Answer from the drawing. Dimensions are ordinates in mm from the lowest x, y and z of the part. A direction names the side the tool comes from. Coordinates: 2 decimals unless noted, no trailing zeros. Write each loop counter-clockwise with the first axis right and the second up, starting at its lowest first coordinate (ties: lowest second). Pieces come first, ordered by that corner, then holes. Notation, with made-up numbers: (17, 16) - (56, 16) arc R16 cw to (56, 31) - close; hole circle Ø1 at (86, 8.5). An arc over 180 degrees is marked (long way). Use one line per item in the form item = value. Start each with the question number.
Item 1: A cutting plane is placed at C-C (y = 24). Write down the section's boundary in (x, z).
Item 2: A cutting plane is placed at D-D (y = 9). Write down the section's boundary in (x, z) (1 decimal).
Item 3: Consider probe 1 along Y at (x, z) = (12.7, 7.5) (1 decimal); probe 2 along Y at (x, z) = (10.25, 24.25); probe 3 along X at (y, z) = (25.4, 6) (1 decimal). Determine where each line is inside the solid, lowest interval first.
Item 4: A cutting plane is placed at A-A (x = 12.7). Write down the section's boundary in (y, z) (1 decimal), then the cut area to 3 significant figures.
Item 5: Determine the mould class of the marked faces 1, 2, 3 and 4 for opening direction Y: released by +Y, released by -Y, zero draft, split by the parting line, or undercut.
Item 6: For the marked faces 5 and 6, determine the directions among +Z, -Z, +X, -X, +Y, -Y from which every point of the face is accessible in a straight line to the end or side of a thin tool.
Item 7: Given pin 1 (5 mm diameter, centred on x = 11, y = 23.5, fed in from +Z); pin 2 (8 mm diameter, centred on x = 19, y = 19, fed in from +Z); pin 3 (10 mm diameter, centred on x = 4, y = 12, fed in from -Z), each flat-ended and moving along its own axis, determine where each tip first touches the part or whether it passes through.
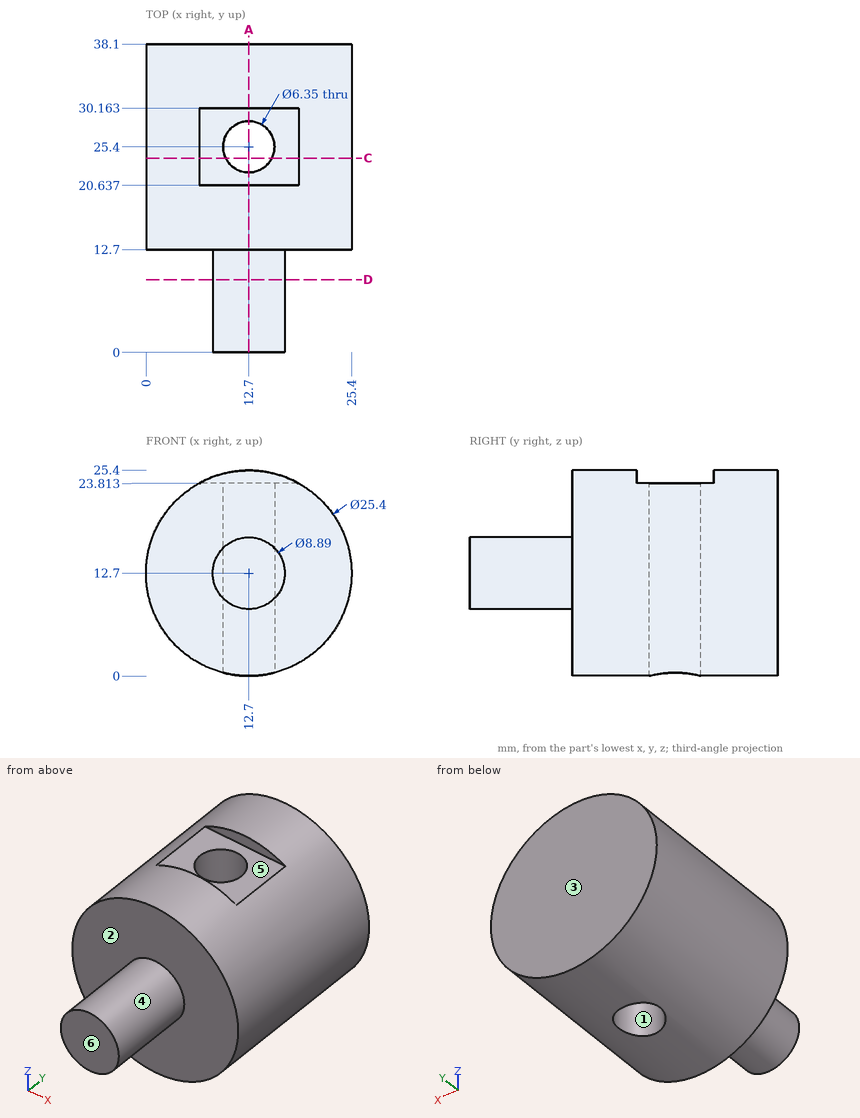
Answer:
q1.outline = (6.55, 23.81) arc R12.7 ccw to (9.85, 0.32) - (9.85, 23.81) - close; (15.55, 0.32) arc R12.7 ccw to (18.85, 23.81) - (15.55, 23.81) - close
q2.outline = circle Ø8.9 at (12.7, 12.7)
q3.probe_1 = 12.7 to 22.2, 28.6 to 38.1
q3.probe_2 = 12.7 to 20.64, 30.16 to 38.1
q3.probe_3 = 1.9 to 9.5, 15.9 to 23.5
q4.outline = (0, 8.3) - (12.7, 8.3) - (12.7, 0) - (22.2, 0) - (22.2, 23.8) - (20.6, 23.8) - (20.6, 25.4) - (12.7, 25.4) - (12.7, 17.1) - (0, 17.1) - close; (28.6, 0) - (38.1, 0) - (38.1, 25.4) - (30.2, 25.4) - (30.2, 23.8) - (28.6, 23.8) - close
q4.area = 592 mm²
q5.face_1 = undercut
q5.face_2 = released by -Y
q5.face_3 = released by +Y
q5.face_4 = zero draft
q6.face_5 = +Z, +X, -X
q6.face_6 = +Z, -Z, +X, -X, -Y
q7.pin_1 = 23.81
q7.pin_2 = 25.19
q7.pin_3 = 0.57
